```python
from build123d import *

# Parameters (mm, degrees)
SKETCH1_W           = 177.8
SKETCH1_H           = 15.24
BOSS_EXTRUDE1_DEPTH = 2.54
SKETCH2_W           = 177.8
SKETCH2_H           = 15.24
SKETCH2_W_2         = 172.72
SKETCH2_H_2         = 10.16
BOSS_EXTRUDE2_DEPTH = 18.796


with BuildPart() as part:
    # Sketch1 → Boss-Extrude1 (new body)
    with BuildSketch(Plane.XY):
        with Locations((88.9, 7.62)):
            Rectangle(SKETCH1_W, SKETCH1_H)
    extrude(amount=BOSS_EXTRUDE1_DEPTH)

    # Sketch2 → Boss-Extrude2 (add)
    with BuildSketch(Plane.XY.offset(2.54)):
        with Locations((88.9, 7.62)):
            Rectangle(SKETCH2_W, SKETCH2_H)
        with Locations((88.9, 7.62)):
            Rectangle(SKETCH2_W_2, SKETCH2_H_2, mode=Mode.SUBTRACT)
    extrude(amount=BOSS_EXTRUDE2_DEPTH)


solid = part.part
```
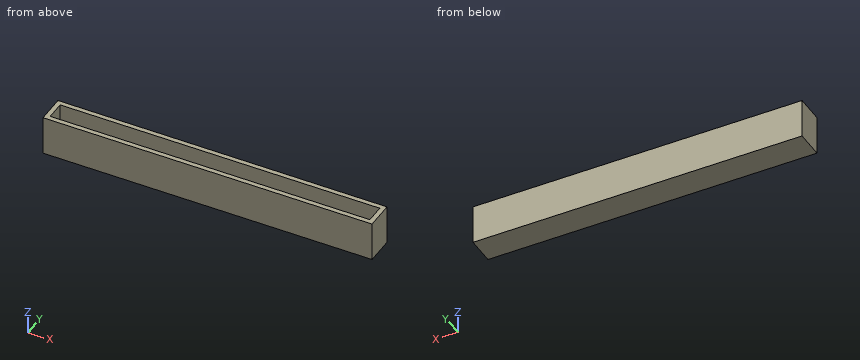
Geometry check sheet. Reference: the model listing, model coordinates, mm. Give positions to 0.01 mm unless a question says otherwise; leave off trailing zeros. Write each loop counter-clockwise with the first axis right and the second up, starting at its lowest first coordinate (ties: lowest second). Pieces come first, ordered by that corner, then holes. Notation, with made-up numbers: (81.25, 33.5) -> (86.25, 33.5) arc R24 cw to (86.25, 55.5) -> close; hole circle Ø6 at (16.5, 68.25). An arc over 180 degrees is marked (long way). Use one line per item in the form item = value.
Item 1: Sectioned sample at A-A on z = 18.25. Enter the section's corners in (x, y), plus the area to 3 significant figures.
Results list:
outline = (0, 0) -> (177.8, 0) -> (177.8, 15.24) -> (0, 15.24) -> close; hole (2.54, 2.54) -> (175.26, 2.54) -> (175.26, 12.7) -> (2.54, 12.7) -> close
area = 955 mm2
Item 2: Scan lines: line 1 (Y direction, x = 14, z = 16.25); line 2 (X direction, y = 10.25, z = 16.25); line 3 (Z direction, x = 113, y = 11.25). Record each from-to range of solid material in increasing order.
Results list:
line_1 = 0 to 2.54, 12.7 to 15.24
line_2 = 0 to 2.54, 175.26 to 177.8
line_3 = 0 to 2.54
Item 3: Sectioned sample at C-C on x = 57. Enter the section's corners in (y, z), plus the area to 3 significant figures.
Results list:
outline = (0, 0) -> (15.24, 0) -> (15.24, 21.34) -> (12.7, 21.34) -> (12.7, 2.54) -> (2.54, 2.54) -> (2.54, 21.34) -> (0, 21.34) -> close
area = 134 mm2
Item 4: Sectioned sample at B-B on y = 8.5. Enter the section's corners in (x, z), plus the area to 3 significant figures.
Results list:
outline = (0, 0) -> (177.8, 0) -> (177.8, 21.34) -> (175.26, 21.34) -> (175.26, 2.54) -> (2.54, 2.54) -> (2.54, 21.34) -> (0, 21.34) -> close
area = 547 mm2
Item 5: Depth check by flat-ended pin: pin 1 Ø5.5 at (x, z) = (68, 7.5) entering from -Y; pin 2 Ø2 at (x, y) = (75, 11) entering from +Z. Enter the tip coordinate at first touch or a pass-through.
Results list:
pin_1 = 0
pin_2 = 2.54
